Model file for the job. Use its own axes, mm. A direction names the side the tool comes from. Give positions to 0.01 mm unless a question says otherwise; leave off trailing zeros. Write each loop counter-clockwise with the first axis right and the second up, starting at its lowest first coordinate (ties: lowest second). Pieces come first, ordered by that corner, then holes. Notation, with made-up numbers: M 72,63.25 L 129,63.25 A23 cw 129,82.25 Z; hole C 85.25,61 d10. An arc over 180 degrees is marked long. Answer as a JSON object with one key per item and string values. Group by question number.
```python
from build123d import *

# Parameters (mm, degrees)
SKETCH002_R        = 25.5
PAD001_DEPTH       = 80.15
PAD006_DEPTH       = 80.15
POLARPATTERN_COUNT = 10
POCKET_DEPTH       = 80.151


with BuildPart() as part:
    # Sketch002 → Pad001 (new body)
    with BuildSketch(Plane.XY):
        Circle(SKETCH002_R)
    extrude(amount=PAD001_DEPTH)

    # Sketch → Pad006 (join)
    with BuildSketch(Plane.XY):
        with BuildLine():
            ThreePointArc((39.721688, -1.5), (39.75, 0), (39.721688, 1.5))
            Line((25.099801, 4.5), (39.721688, 1.5))
            Line((25.099801, 4.5), (17, 0))
            Line((17, 0), (25.099801, -4.5))
            Line((25.099801, -4.5), (39.721688, -1.5))
        make_face()
    pad006 = extrude(amount=PAD006_DEPTH)

    # PolarPattern: Pad006 ×10 about axis
    polarpattern_axis = Axis((0, 0, 0), (0, 0, 1))
    for i in range(1, POLARPATTERN_COUNT):
        add(pad006.rotate(polarpattern_axis, i * 360 / POLARPATTERN_COUNT))

    # Sketch001 → Pocket (cut, through all)
    with BuildSketch(Plane.XY):
        Polygon((14.3875, 8.306627), (0, 16.613254), (-14.3875, 8.306627), (-14.3875, -8.306627), (0, -16.613254), (14.3875, -8.306627), align=None)
    extrude(amount=POCKET_DEPTH, mode=Mode.SUBTRACT)


with BuildPart() as part_1:
    # Body027 placement: moved
    add(part.part.moved(Location((0, -100, 0))))


solid = part_1.part
```
Q1. 3-axis set-ups, long thin cutter, end or side, ignore diameter. For faces 4 (the flat face through (-27.914, -116.546, 39.514)), 5 (the flat face through (7.09, -112.52, 39.51)), 6 (the flat face through (7.11, -131.66, 39.51)): which of +Z, -Z, +X, -X, +Y, -Y reach the whole face in a straight line?
Q2. Slice it at A-A, the plane y = -79. Write the cut outline in (x, z).
Q3. Slice it at B-B, the plane x = -8.5. Write the cut outline in (y, z), then the cut area to 3 significant figures.
Q4. Slice it at D-D, the plane x = 27. Write the cut outline in (y, z), then the cut area to 3 significant figures.
Q5. Slice it at C-C, the plane y = -114.5. Write the cut outline in (x, z), then the cut area to 3 significant figures.
Q6. Two-plate mould, pull along Y, no slides. Class faces 1 (the flat face through (32.31, -96.98, 39.51)), 2 (the flat face through (-7.11, -68.34, 39.51)), 3 (the flat face through (-24.362, -121.434, 39.514)): +Y half, -Y half, draft (parallel to the pull), parting line (faces both ways), or undercut.
Q7. Wall check: L1, parallel to X at y = -78, z = 6; L2, parallel to X at y = -120, z = 75.5; L3, parallel to X at y = -69, z = 32. Give the ranges that are in metal, low to high.
Q8. Drop flat-ended pins along their axis: P1, Ø18.5, axis at y = -98, z = 30.5, coming from the -X side; P2, Ø1.5, axis at y = -116.5, z = 50.5, coming from the +X side; P3, Ø8, axis at x = 5, z = 64.5, coming from the +Y side. Give the stop position or say it passes through.
Solved:
{
 "1": {"face 4": "+Z, -Z, -X", "face 5": "+Z, -Z", "face 6": "+Z, -Z, -Y"},
 "2": {"outline": "M -31.98,0 L -23.4,0 L -23.4,80.15 L -31.98,80.15 Z; M -14.47,0 L 14.47,0 L 14.47,80.15 L -14.47,80.15 Z; M 23.4,0 L 31.98,0 L 31.98,80.15 L 23.4,80.15 Z"},
 "3": {"outline": "M -134.11,0 L -111.71,0 L -111.71,80.15 L -134.11,80.15 Z; M -88.29,0 L -65.89,0 L -65.89,80.15 L -88.29,80.15 Z", "area": "3,590 mm²"},
 "4": {"outline": "M -122.63,0 L -115.55,0 L -115.55,80.15 L -122.63,80.15 Z; M -104.11,0 L -95.89,0 L -95.89,80.15 L -104.11,80.15 Z; M -84.45,0 L -77.37,0 L -77.37,80.15 L -84.45,80.15 Z", "area": "1,790 mm²"},
 "5": {"outline": "M -26.04,0 L -3.66,0 L -3.66,80.15 L -26.04,80.15 Z; M 3.66,0 L 26.04,0 L 26.04,80.15 L 3.66,80.15 Z", "area": "3,590 mm²"},
 "6": {"face 1": "undercut", "face 2": "+Y half", "face 3": "-Y half"},
 "7": {"L1": "x = -32.89 to -25.61, -12.89 to 12.89, 25.61 to 32.89", "L2": "x = -31.07 to -21.2, -15.82 to 15.82, 21.2 to 31.07", "L3": "x = -12.99 to -6.74, 6.74 to 12.99"},
 "8": {"P1": "stops at x = -39.75", "P2": "stops at x = 28.56", "P3": "stops at y = -65.01"}
}
